Autodesk Inventor part; units mm, degrees
ref_plane "YZ Plane" through (0, 0, 0) normal (1, 0, 0) x (0, 1, 0)
ref_plane "XZ Plane" through (0, 0, 0) normal (0, 1, 0) x (-1, 0, 0)
ref_plane "XY Plane" through (0, 0, 0) normal (0, 0, 1) x (1, 0, 0)
sketch "Sketch1" plane through (0, 0, 0) normal (0, 1, 0) x (-1, 0, 0)
  line L0 (4.7625, -9.525) -> (-4.7625, -9.525)
  line L1 (-4.7625, -9.525) -> (-4.7625, 9.525)
  line L2 (-4.7625, 9.525) -> (4.7625, 9.525)
  line L3 (4.7625, 9.525) -> (4.7625, -9.525)
  line L4 (5.7625, -10.525) -> (-5.7625, -10.525)
  line L5 (-5.7625, -10.525) -> (-5.7625, 10.525)
  line L6 (-5.7625, 10.525) -> (5.7625, 10.525)
  line L7 (5.7625, 10.525) -> (5.7625, -10.525)
  point P0 (0, 0)
  dimension "d0" = 19.05
  dimension "d1" = 21.05
  dimension "d2" = 9.525
  dimension "d3" = 10.525
  dimension "d4" = 9.525
  dimension "d5" = 4.7625
  dimension "d6" = 11.525
  dimension "d7" = 5.7625
extrude "Extrusion1" add sketch "Sketch1" against normal blind 142
sketch "Sketch2" plane through (5.7625, 0, -10.525) normal (0, 0, -1) x (-1, 0, 0)
  line L0 (11.525, 0) -> (0, 0)
  line L1 (0, 0) -> (0, -142)
  line L2 (11.525, 0) -> (11.525, -142)
  line L3 (-7.7677, -71) -> (26.0331, -71) construction
  line L4 (10.525, -73.9) -> (1, -73.9)
  line L5 (1, -73.9) -> (1, -68.1)
  line L6 (1, -68.1) -> (10.525, -68.1)
  line L7 (10.525, -68.1) -> (10.525, -73.9)
  line L8 (10.525, -67.85) -> (1, -67.85)
  line L9 (1, -67.85) -> (1, -62.05)
  line L10 (1, -62.05) -> (10.525, -62.05)
  line L11 (10.525, -62.05) -> (10.525, -67.85)
  line L12 (10.525, -61.8) -> (1, -61.8)
  line L13 (1, -61.8) -> (1, -56)
  line L14 (1, -56) -> (10.525, -56)
  line L15 (10.525, -56) -> (10.525, -61.8)
  line L16 (10.525, -74.15) -> (1, -74.15)
  line L17 (1, -74.15) -> (1, -79.95)
  line L18 (1, -79.95) -> (10.525, -79.95)
  line L19 (10.525, -79.95) -> (10.525, -74.15)
  line L20 (10.525, -80.2) -> (1, -80.2)
  line L21 (1, -80.2) -> (1, -86)
  line L22 (1, -86) -> (10.525, -86)
  line L23 (10.525, -86) -> (10.525, -80.2)
  point P0 (5.7625, 0)
  dimension "d12" = 71
  dimension "d13" = 5.8
  dimension "d14" = 2.9
  dimension "d15" = 5.8
  dimension "d16" = 5.8
  dimension "d17" = 0.25
  dimension "d18" = 0.25
  dimension "d19" = 5.8
  dimension "d20" = 5.8
  dimension "d25" = 0.25
  dimension "d26" = 0.25
  dimension "d27" = 1
  dimension "d28" = 1
  dimension "d29" = 1
  dimension "d30" = 1
  dimension "d31" = 1
  dimension "d32" = 1
  dimension "d33" = 1
  dimension "d34" = 1
  dimension "d35" = 1
  dimension "d36" = 1
extrude "Extrusion2" cut sketch "Sketch2" against normal through all
equation "\"d14\" = 0.5 * d13"
equation "\"d15\" = d13"
equation "\"d16\" = d13"
equation "\"d19\" = d13"
equation "\"d20\" = d13"
equation "\"d28\" = d27"
equation "\"d29\" = d27"
equation "\"d30\" = d27"
equation "\"d31\" = d27"
equation "\"d32\" = d27"
equation "\"d33\" = d27"
equation "\"d34\" = d27"
equation "\"d35\" = d27"
equation "\"d36\" = d27"
properties part number "Waveguide"
The listing builds one solid part. Answer for the finished solid, in the listing's coordinates (mm). A direction names the side the tool comes from. Give positions to 0.01 mm unless a question says otherwise; leave off trailing zeros. Write each loop counter-clockwise with the first axis right and the second up, starting at its lowest first coordinate (ties: lowest second). Pieces come first, ordered by that corner, then holes. Notation, with made-up numbers: (71.25, 22.25) - (92.25, 22.25) arc R24 ccw to (92.25, 53.25) - close; hole circle Ø9 at (89.5, 27.25). An arc over 180 degrees is marked (long way). Use one line per item in the form item = value. Start each with the question number.
1) Find section D-D on x = 0. Count the separate pieces of the cut face and the enclosed holes in it, plus the area to 3 significant figures.
2) Find section C-C on y = -42.5. Determine the outline of the cut face in (x, z) (1 decimal).
3) A tool of negligible diameter and unlimited length cuts with its end or side. For faces 4 (the face through (0, -114, 9.525)), 5 (the face through (-5.762, -70, 0)), from which of +Z, -Z, +X, -X, +Y, -Y can it reach the whole face along a straight path? Write none if from no direction.
4) Find section A-A on z = 3. Determine the outline of the cut face in (x, y), plus the area to 3 significant figures.
5) A flat-ended cylindrical pin translates along its axis: pin 1 Ø0.8 at (x, z) = (-1.5, -10) entering from +Y. Find the tip coordinate at first contact, or state that the pin passes through.
6) Find section B-B on y = -77. Determine the outline of the cut face in (x, z) (1 decimal), plus the area to 3 significant figures.
7) The mould has two halves that part along Z. Classify faces 1 (the face through (5, 0, 1)), 2 (the face through (-5, -70, 10.525)), 3 (the face through (-4.762, -72, 0)): pulls with the +Z half, pulls with the -Z half, needs draft (parallel to the pull), parting line crosses it, or undercut.
8) Consider line 1 along Z through (x, y) = (-2.25, -36) (3 decimals); line 2 along X through (y, z) = (-20.5, -2.75). Determine where each line is inside the solid, lowest interval first. Write a range as from..to.
Geometry results:
q1.separate_pieces = 12
q1.enclosed_holes = 0
q1.area = 226 mm2
q2.outline = (-5.8, -10.5) - (5.8, -10.5) - (5.8, 10.5) - (-5.8, 10.5) - close; hole (-4.8, -9.5) - (4.8, -9.5) - (4.8, 9.5) - (-4.8, 9.5) - close
q3.face_4 = +Y, -Y
q3.face_5 = +Z, -Z, -X, +Y, -Y
q4.outline = (-5.76, -142) - (-4.76, -142) - (-4.76, 0) - (-5.76, 0) - close; (4.76, -142) - (5.76, -142) - (5.76, 0) - (4.76, 0) - close
q4.area = 284 mm2
q5.pin_1 = 0
q6.outline = (-5.8, -10.5) - (-4.8, -10.5) - (-4.8, 10.5) - (-5.8, 10.5) - close; (4.8, -10.5) - (5.8, -10.5) - (5.8, 10.5) - (4.8, 10.5) - close
q6.area = 42.1 mm2
q7.face_1 = needs draft
q7.face_2 = pulls with the +Z half
q7.face_3 = undercut
q8.line_1 = -10.525..-9.525, 9.525..10.525
q8.line_2 = -5.76..-4.76, 4.76..5.76
